from build123d import *

# Parameters (mm, degrees)
F0_R     = 76.385424
F1_DEPTH = 228.6
F2_R     = 52.72962
F3_DEPTH = 14.478
F4_R     = 65.606028
F5_DEPTH = 25.4
F6_R     = 10.679564
F7_DEPTH = 21.082
F8_R     = 6.299562
F9_DEPTH = 13.716


with BuildPart() as f1:
    # F0 (on Top) → F1 (new body)
    with BuildSketch(Plane.XY):
        Circle(F0_R)
    extrude(amount=F1_DEPTH)

    # F2 (on face) → F3 (join)
    with BuildSketch(Plane.XY.offset(228.6)):
        Circle(F2_R)
    extrude(amount=F3_DEPTH)

    # F4 (on face) → F5 (join)
    with BuildSketch(Plane.XY.offset(243.078)):
        Circle(F4_R)
    extrude(amount=F5_DEPTH)

    # F6 (on face) → F7 (join)
    with BuildSketch(Plane(origin=(0, 0, 0), x_dir=(1, 0, 0), z_dir=(0, 0, -1))):
        Circle(F6_R)
    extrude(amount=F7_DEPTH)

    # F8 (on face) → F9 (join)
    with BuildSketch(Plane(origin=(0, 0, -21.082), x_dir=(1, 0, 0), z_dir=(0, 0, -1))):
        Circle(F8_R)
    extrude(amount=F9_DEPTH)


solid = f1.part
The model under review builds one solid part; all positions refer to its coordinate system, in mm. A direction names the side the tool comes from. Give positions to 0.01 mm unless a question says otherwise; leave off trailing zeros. Write each loop counter-clockwise with the first axis right and the second up, starting at its lowest first coordinate (ties: lowest second). Pieces come first, ordered by that corner, then holes.
1. Add section A-A, the plane x = 0. Write out the cut boundary in (y, z), plus the area to 3 significant figures.
2. Draft analysis for pull direction Z (two halves, no side actions). For faces 1 (the flat face through (-1, 1, 268.478)), 2 (the flat face through (0, 54, 243.078)), 3 (the cylindrical face through (-60.6, -46.5, 112.7)), state which applies: +Z half, -Z half, draft (parallel to the pull), parting line (faces both ways), or undercut.
3. For P1, Ø3, axis at x = 36, z = 136, coming from the +Y side; P2, Ø8, axis at x = -58.5, z = 177, coming from the -Y side; P3, Ø1, axis at x = -48.5, z = 134, coming from the -Y side, all flat-tipped, find the tip position at first contact; note any pin that passes through.
4. Add section B-B, the plane y = 60. Write out the cut boundary in (x, z).
5. Tool access review of faces 4 (the cylindrical face through (-14.222, -64.046, 255.6)), 5 (the flat face through (0, 0, -34.798)), 6 (the flat face through (-18, -50, 228.6)), 7 (the cylindrical face through (10.186, -3.208, -10.393)): name each direction out of +Z, -Z, +X, -X, +Y, -Y from which nothing blocks a thin tool from reaching the whole face with its end or side.
6. Wall thickness on L1, parallel to Z at x = -49, y = 30; L2, parallel to Z at x = -44.5, y = -9.5; L3, parallel to Z at x = 26.5, y = -66.5: over which ranges is each line inside the solid? List them lowest first.
7. Add section D-D, the plane x = 56.5. Write out the cut boundary in (y, z), plus the area to 3 significant figures.
Worked answers:
1. outline: (-76.39, 0) - (-10.68, 0) - (-10.68, -21.08) - (-6.3, -21.08) - (-6.3, -34.8) - (6.3, -34.8) - (6.3, -21.08) - (10.68, -21.08) - (10.68, 0) - (76.39, 0) - (76.39, 228.6) - (52.73, 228.6) - (52.73, 243.08) - (65.61, 243.08) - (65.61, 268.48) - (-65.61, 268.48) - (-65.61, 243.08) - (-52.73, 243.08) - (-52.73, 228.6) - (-76.39, 228.6) - close
1. area: 40,400 mm2
2. face 1: +Z half
2. face 2: undercut
2. face 3: draft
3. P1: stops at y = 68.15
3. P2: stops at y = -53.52
3. P3: stops at y = -59.42
4. outline: (-47.27, 0) - (47.27, 0) - (47.27, 228.6) - (-47.27, 228.6) - close; (-26.54, 243.08) - (26.54, 243.08) - (26.54, 268.48) - (-26.54, 268.48) - close
5. face 4: +Z
5. face 5: -Z, +X, -X, +Y, -Y
5. face 6: none
5. face 7: -Z
6. L1: z = 0 to 228.6, 243.08 to 268.48
6. L2: z = 0 to 268.48
6. L3: z = 0 to 228.6
7. outline: (-51.41, 0) - (51.41, 0) - (51.41, 228.6) - (-51.41, 228.6) - close; (-33.35, 243.08) - (33.35, 243.08) - (33.35, 268.48) - (-33.35, 268.48) - close
7. area: 25,200 mm2
